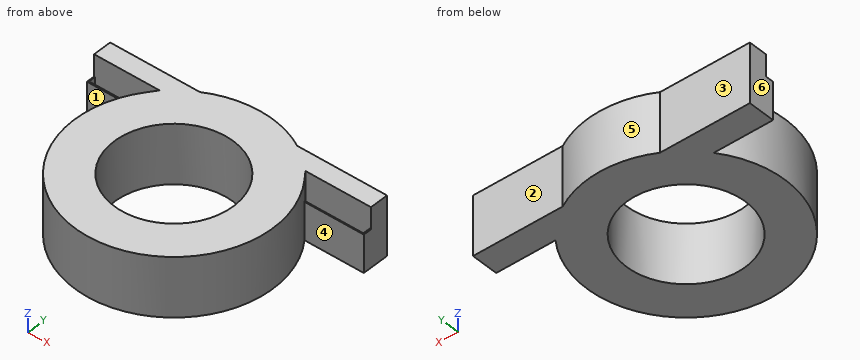
```python
from build123d import *

# Parameters (mm, degrees)
F1_DEPTH = 38.1
F3_DEPTH = 25.4
F5_DEPTH = 11.43


with BuildPart() as f1:
    # F0 (on Top) → F1 (new body)
    with BuildSketch(Plane.XY):
        with BuildLine():
            ThreePointArc((-50.8, 38.1), (-20.0804631421, -60.2413894262), (63.5, 0))
            ThreePointArc((63.5, 0), (60.2413894262, 20.0804631421), (50.8, 38.1))
            Line((50.8, 38.1), (0, 38.1))
            Line((0, 38.1), (-50.8, 38.1))
        make_face()
        with BuildLine():
            ThreePointArc((38.1, 0), (-26.9407683632, -26.9407683632), (0, 38.1))
            ThreePointArc((0, 38.1), (26.9407683632, 26.9407683632), (38.1, 0))
        make_face(mode=Mode.SUBTRACT)
        with BuildLine():
            Line((0, 38.1), (50.8, 38.1))
            ThreePointArc((50.8, 38.1), (41.9294068416, 47.6883092792), (31.2845870641, 55.258706212))
            Line((31.2845870641, 55.258706212), (0, 55.258706212))
            Line((0, 55.258706212), (0, 38.1))
        make_face()
        with BuildLine():
            ThreePointArc((31.2845870641, 55.258706212), (41.9294068416, 47.6883092792), (50.8, 38.1))
            Line((50.8, 38.1), (88.9, 38.1))
            Line((88.9, 38.1), (88.9, 55.258706212))
            Line((88.9, 55.258706212), (31.2845870641, 55.258706212))
        make_face()
        with BuildLine():
            Line((-88.9, 38.1), (-50.8, 38.1))
            ThreePointArc((-50.8, 38.1), (-41.9294068416, 47.6883092792), (-31.2845870641, 55.258706212))
            Line((-31.2845870641, 55.258706212), (-88.9, 55.258706212))
            Line((-88.9, 55.258706212), (-88.9, 38.1))
        make_face()
        with BuildLine():
            ThreePointArc((-31.2845870641, 55.258706212), (-41.9294068416, 47.6883092792), (-50.8, 38.1))
            Line((-50.8, 38.1), (0, 38.1))
            Line((0, 38.1), (0, 55.258706212))
            Line((0, 55.258706212), (-31.2845870641, 55.258706212))
        make_face()
        with BuildLine():
            Line((0, 55.258706212), (31.2845870641, 55.258706212))
            ThreePointArc((31.2845870641, 55.258706212), (0, 63.5), (-31.2845870641, 55.258706212))
            Line((-31.2845870641, 55.258706212), (0, 55.258706212))
        make_face()
    extrude(amount=F1_DEPTH)

    # F2 (on face) → F3 (cut)
    with BuildSketch(Plane.XY.offset(38.1)):
        Polygon((-46.8710027635, 43.4018671513), (-88.9, 43.4018671513), (-88.9, 38.1), (-50.8, 38.1), align=None)
        Polygon((88.9, 38.1), (88.9, 43.4018671513), (46.863, 43.4018671513), (50.8, 38.1), align=None)
    extrude(amount=-F3_DEPTH, mode=Mode.SUBTRACT)

    # F4 (on face) → F5 (join)
    with BuildSketch(Plane.XY.offset(12.7)):
        Polygon((-50.1407290747, 38.9896333218), (-88.2961526513, 38.9896333218), (-88.2961526513, 43.4018671513), (-88.9, 43.4018671513), (-88.9, 38.9896333218), (-88.9, 38.1), (-50.8, 38.1), align=None)
        Polygon((88.9, 38.1), (88.9, 43.4018671513), (88.0254730582, 43.4018671513), (88.0254730582, 38.7667292968), (50.304907768, 38.7667292968), (50.8, 38.1), align=None)
    extrude(amount=F5_DEPTH)


solid = f1.part
```
Geometry check sheet. Reference: the model listing, model coordinates, mm. Face numbers are marked on the shaded views. A direction names the side the tool comes from. Round coordinates to 2 decimals unless told otherwise and drop trailing zeros. Loops run counter-clockwise (first coordinate to the right, second up) from the corner with the lowest first, then second, coordinate; pieces in that order, holes last. Notation, with made-up numbers: (75.5, 32.5) - (131.5, 32.5) arc R11 ccw to (131.5, 38.5) - close; hole circle Ø1 at (-11, 23). An arc over 180 degrees is marked (long way). Use a Markdown table: item, result.
Q1. Cross-section at B-B on z = 28. Record the cut outline in (x, y), plus the area to 3 significant figures.
Solutions:
| item | result |
|---|---|
| outline | (-88.9, 43.4) - (-46.87, 43.4) - (-50.8, 38.1) arc R63.5 ccw (long way) to (50.8, 38.1) - (46.86, 43.4) - (88.9, 43.4) - (88.9, 55.26) - (31.28, 55.26) arc R63.5 ccw to (-31.28, 55.26) - (-88.9, 55.26) - close; hole circle Ø76.2 at (0, 0) |
| area | 9,280 mm2 |
Q2. Access from +Z, -Z, +X, -X, +Y, -Y to the whole of each face (thin tool, end or side, straight path). Record for the marked faces 1, 2 and 3.
Solutions:
| item | result |
|---|---|
| face 1 | +Z, -Z, -X |
| face 2 | +Z, -Z, +X, +Y |
| face 3 | +Z, -Z, -X, +Y |
Q3. Material ranges on line 1 (X direction, y = 0, z = 8.5); line 2 (Y direction, x = 80, z = 30.5); line 3 (Y direction, x = -54, z = 33.5), recorded low to high.
Solutions:
| item | result |
|---|---|
| line 1 | x = -63.5 to -38.1, 38.1 to 63.5 |
| line 2 | y = 43.4 to 55.26 |
| line 3 | y = -33.41 to 33.41, 43.4 to 55.26 |
Q4. Go/stop test with flat-tipped pins: P1, Ø12.5, axis at x = -69, z = 16.5, coming from the +Y side; P2, Ø12.5, axis at x = -64, z = 25, coming from the -Y side; P3, Ø5, axis at y = -36, z = 31.5, coming from the +X side. Record where each tip stops, or that it passes through.
Solutions:
| item | result |
|---|---|
| P1 | stops at y = 55.26 |
| P2 | stops at y = -26.4 |
| P3 | stops at x = 53.94 |
Q5. Draft check along Y on the marked faces 4, 5 and 6. Enter one of: released by +Y, released by -Y, zero draft, split by the parting line, or undercut.
Solutions:
| item | result |
|---|---|
| face 4 | undercut |
| face 5 | released by +Y |
| face 6 | zero draft |
Q6. Cross-section at D-D on z = 14.5. Record the cut outline in (x, y).
Solutions:
| item | result |
|---|---|
| outline | (-88.9, 38.1) - (-50.8, 38.1) arc R63.5 ccw (long way) to (50.8, 38.1) - (88.9, 38.1) - (88.9, 55.26) - (31.28, 55.26) arc R63.5 ccw to (-31.28, 55.26) - (-88.9, 55.26) - close; hole (-88.3, 38.99) - (-50.14, 38.99) - (-46.87, 43.4) - (-88.3, 43.4) - close; hole circle Ø76.2 at (0, 0); hole (46.86, 43.4) - (50.3, 38.77) - (88.03, 38.77) - (88.03, 43.4) - close |
Q7. Cross-section at A-A on y = 0. Record the cut outline in (x, z), plus the area to 3 significant figures.
Solutions:
| item | result |
|---|---|
| outline | (-63.5, 0) - (-38.1, 0) - (-38.1, 38.1) - (-63.5, 38.1) - close; (38.1, 0) - (63.5, 0) - (63.5, 38.1) - (38.1, 38.1) - close |
| area | 1,940 mm2 |
